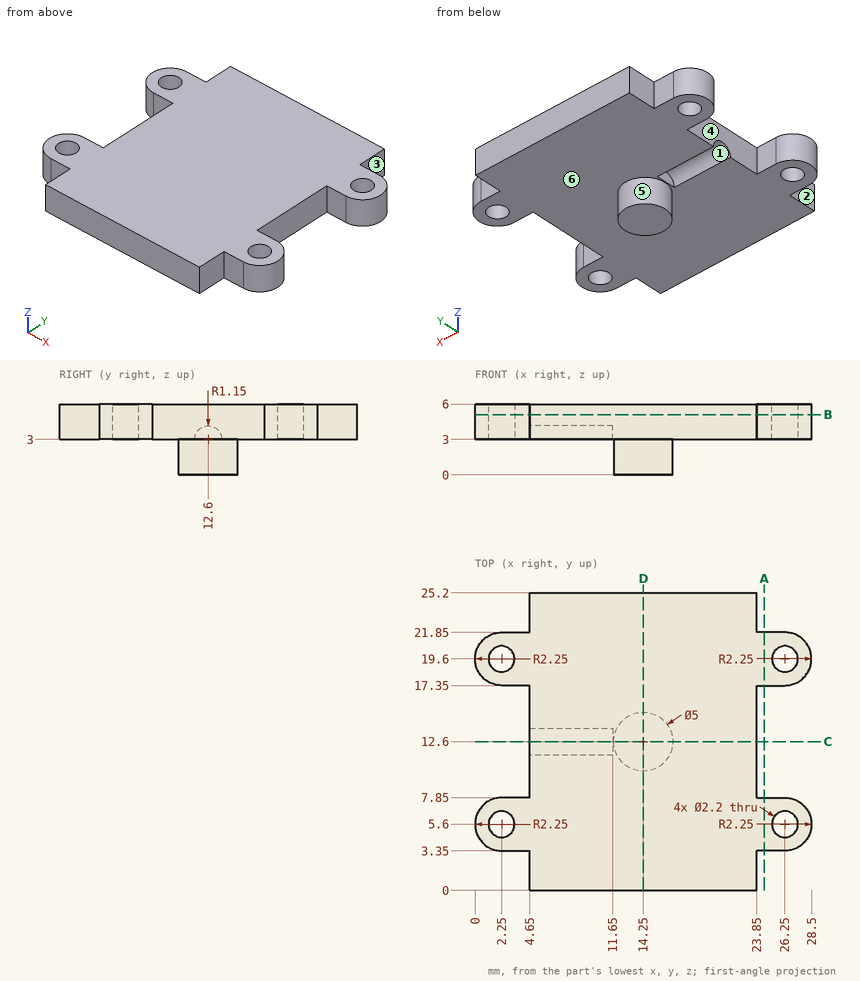
Answer from the drawing. Dimensions are ordinates in mm from the lowest x, y and z of the part. A direction names the side the tool comes from. Coordinates: 2 decimals unless noted, no trailing zeros. Write each loop counter-clockwise with the first axis right and the second up, starting at its lowest first coordinate (ties: lowest second). Pieces come first, ordered by that corner, then holes. Notation, with made-up numbers: (37, 46.25) - (72, 46.25) arc R19 cw to (72, 82.25) - close; hole circle Ø11 at (19.25, 9). An arc over 180 degrees is marked (long way). Return JSON: item names as keys, results as strings.
1. The part is cut by section A-A on x = 24.5. Determine the outline of the cut face in (y, z).
Final values:
{"outline": "(3.35, 3) - (7.85, 3) - (7.85, 6) - (3.35, 6) - close; (17.35, 3) - (21.85, 3) - (21.85, 6) - (17.35, 6) - close"}
2. The part is cut by section B-B on z = 5.1. Determine the outline of the cut face in (x, y).
Final values:
{"outline": "(2.25, 3.35) - (4.65, 3.35) - (4.65, 0) - (23.85, 0) - (23.85, 3.35) - (26.25, 3.35) arc R2.25 ccw to (26.25, 7.85) - (23.85, 7.85) - (23.85, 17.35) - (26.25, 17.35) arc R2.25 ccw to (26.25, 21.85) - (23.85, 21.85) - (23.85, 25.2) - (4.65, 25.2) - (4.65, 21.85) - (2.25, 21.85) arc R2.25 ccw to (2.25, 17.35) - (4.65, 17.35) - (4.65, 7.85) - (2.25, 7.85) arc R2.25 ccw to start; hole circle Ø2.2 at (2.25, 5.6); hole circle Ø2.2 at (2.25, 19.6); hole circle Ø2.2 at (26.25, 5.6); hole circle Ø2.2 at (26.25, 19.6)"}
3. The part is cut by section C-C on y = 12.6. Determine the outline of the cut face in (x, z).
Final values:
{"outline": "(4.65, 4.15) - (11.65, 4.15) - (11.65, 3) - (11.75, 3) - (11.75, 0) - (16.75, 0) - (16.75, 3) - (23.85, 3) - (23.85, 6) - (4.65, 6) - close"}
4. For a pull along Y with two mould halves and no side action, classify the marked faces 4, 5 and 6 as +Y half, -Y half, draft (parallel to the pull), parting line (faces both ways), or undercut.
Final values:
{"face 4": "undercut", "face 5": "parting line", "face 6": "draft"}
5. The part is cut by section D-D on x = 14.25. Determine the outline of the cut face in (y, z).
Final values:
{"outline": "(0, 3) - (10.1, 3) - (10.1, 0) - (15.1, 0) - (15.1, 3) - (25.2, 3) - (25.2, 6) - (0, 6) - close"}
6. Which of the six approach directions +Z, -Z, +X, -X, +Y, -Y give full straight-line access (tool end or side, diameter ignored) to the marked faces 1, 2 and 3?
Final values:
{"face 1": "-Z, -X", "face 2": "+Z, -Z, -X, -Y", "face 3": "+Z, -Z, +X, +Y"}
7. Consider line 1 along Y through (x, z) = (26.25, 5.2); line 2 along X through (y, z) = (19.6, 4.3); line 3 along Y through (x, z) = (25, 5.1). Determine where each line is inside the solid, lowest interval first.
Final values:
{"line 1": "3.35 to 4.5, 6.7 to 7.85, 17.35 to 18.5, 20.7 to 21.85", "line 2": "0 to 1.15, 3.35 to 25.15, 27.35 to 28.5", "line 3": "3.35 to 7.85, 17.35 to 21.85"}
8. Each of these flat-tipped pins is pushed along its axis until it touches: pin 1 Ø1.2 at (x, z) = (3, 4) entering from -Y; pin 2 Ø3.5 at (x, y) = (2.25, 19.6) entering from -Z; pin 3 Ø0.9 at (y, z) = (23, 5) entering from -X; pin 4 Ø2.5 at (x, z) = (4, 4) entering from +Y. Where does it stop, or does it pass through?
Final values:
{"pin 1": "y = 3.35", "pin 2": "z = 3", "pin 3": "x = 4.65", "pin 4": "y = 25.2"}
